Geometry check sheet. Reference: the model listing, model coordinates, mm. A direction names the side the tool comes from. Round coordinates to 2 decimals unless told otherwise and drop trailing zeros. Write each loop counter-clockwise with the first axis right and the second up, starting at its lowest first coordinate (ties: lowest second). Pieces come first, ordered by that corner, then holes. Notation, with made-up numbers: M -10,53 L 37,53 A27 ccw 37,86 Z; hole C -7,31.25 d9. An arc over 180 degrees is marked long. One line per item, written item: value. Start each with the question number.
1. Section check D-D (y = -2). Record the boundary of the cut face in (x, z).
2. Release check for a two-part mould opening along Z. For faces 1 (the flat face through (32, -2, 33)), 2 (the flat face through (41, -28.6, 17)), 3 (the flat face through (1.479, -19.529, 12.122)) record: pulls with the +Z half, pulls with the -Z half, needs draft (parallel to the pull), parting line crosses it, or undercut.
3. Access from +Z, -Z, +X, -X, +Y, -Y to the whole of each face (thin tool, end or side, straight path). Record for faces 4 (the flat face through (0, -21, 13)), 5 (the flat face through (54, -22.6, 17)), 6 (the flat face through (1.479, -8.922, 12.271)), 7 (the flat face through (65, -5, 17)).
4. Section check B-B (z = 29). Record the boundary of the cut face in (x, y).
5. Section check C-C (x = 47). Record the boundary of the cut face in (y, z), and give its area (3 significant figures).
6. Depth check by flat-ended pin: P1, Ø3, axis at y = -14.3, z = 17.5, coming from the +X side; P2, Ø6, axis at y = -17.5, z = 7.5, coming from the +X side; P3, Ø3, axis at y = -3.5, z = 27.5, coming from the +X side. Enter the tip coordinate at first touch or a pass-through.
7. Section check A-A (x = 7). Record the boundary of the cut face in (y, z), and give its area (3 significant figures).
8. Scan lines: probe 1 along Z at (x, y) = (9.25, -14.3); probe 2 along Y at (x, z) = (32.5, 29); probe 3 along X at (y, z) = (-19.5, 26.5). Record each from-to range of solid material in increasing order. Write a range as [from, to].
from build123d import *

# Parameters (mm, degrees)
EXTRUDE_1_DEPTH     = 35
CUT_EXTRUDE_2_DEPTH = 3
SKETCH_4_R          = 2.5
CUT_EXTRUDE_3_DEPTH = 15
CHAMFER_2_SIZE      = 4
CHAMFER_3_SIZE      = 4
CHAMFER_4_SIZE      = 4
CHAMFER_4_SIZE2     = 15
CHAMFER_5_SIZE      = 15
CHAMFER_5_SIZE2     = 4


with BuildPart() as part:
    # Эскиз2 → Бобышка-Вытянуть1 (new body)
    with BuildSketch(Plane.XY):
        Polygon((0, 0), (65, 0), (65, -6), (15, -6), (15, -22.6), (95, -22.6), (95, -28.6), (0, -28.6), align=None)
    extrude(amount=EXTRUDE_1_DEPTH)

    # Эскиз3 → Вырез-Вытянуть2 (cut)
    with BuildSketch(Plane.ZY):
        Polygon((6.893398282, -14.3), (17.5, -24.906601718), (28.106601718, -14.3), (17.5, -3.693398282), align=None)
    extrude(amount=-CUT_EXTRUDE_2_DEPTH, mode=Mode.SUBTRACT)

    # Эскиз4 → Вырез-Вытянуть3 (cut)
    with BuildSketch(Plane.ZY):
        with Locations(Location((17.5, -14.3, 0), (0, 0, 270))):
            Circle(SKETCH_4_R)
    extrude(amount=-CUT_EXTRUDE_3_DEPTH, mode=Mode.SUBTRACT)

    # Фаска2
    chamfer_2_edges = [part.edges().sort_by_distance(p)[0] for p in [
        (15, -11.8, 17.5),
    ]]
    chamfer(chamfer_2_edges, length=CHAMFER_2_SIZE)

    # Фаска3
    chamfer_3_edges = [part.edges().sort_by_distance(p)[0] for p in [
        (47.5, -28.6, 0),
        (32.5, 0, 35),
        (32.5, 0, 0),
        (47.5, -28.6, 35),
    ]]
    chamfer(chamfer_3_edges, length=CHAMFER_3_SIZE)

    # Фаска4
    chamfer_4_edges = [part.edges().sort_by_distance(p)[0] for p in [
        (65, 0, 17.5),
    ]]
    chamfer_4_side = [part.faces().sort_by_distance(p)[0] for p in [
        (65, -3.137457045, 17.5),
    ]]
    chamfer(chamfer_4_edges, length=CHAMFER_4_SIZE, length2=CHAMFER_4_SIZE2, reference=chamfer_4_side[0])

    # Фаска5
    chamfer_5_edges = [part.edges().sort_by_distance(p)[0] for p in [
        (95, -28.6, 17.5),
    ]]
    chamfer_5_side = [part.faces().sort_by_distance(p)[0] for p in [
        (47.5, -28.6, 17.5),
    ]]
    chamfer(chamfer_5_edges, length=CHAMFER_5_SIZE, length2=CHAMFER_5_SIZE2, reference=chamfer_5_side[0])


solid = part.part
Result sheet:
1. outline: M 0,2 L 57.5,2 L 57.5,33 L 0,33 Z
2. face 1: pulls with the +Z half
2. face 2: needs draft
2. face 3: undercut
3. face 4: +Z, -Z, -X, +Y, -Y
3. face 5: +Z, -Z, +X
3. face 6: -X
3. face 7: +Z, -Z, +X, +Y
4. outline: M 0,-28.6 L 80,-28.6 L 95,-24.6 L 95,-22.6 L 15,-22.6 L 15,-6 L 65,-6 L 65,-4 L 50,0 L 0,0 Z
5. outline: M -28.6,4 L -24.6,0 L -22.6,0 L -22.6,35 L -24.6,35 L -28.6,31 Z; M -6,0 L -4,0 L 0,4 L 0,31 L -4,35 L -6,35 Z
5. area: 388 mm2
6. P1: passes through
6. P2: stops at x = 15
6. P3: stops at x = 65
7. outline: M -28.6,4 L -24.6,0 L -4,0 L 0,4 L 0,31 L -4,35 L -24.6,35 L -28.6,31 Z; hole C -14.3,17.5 d5
7. area: 949 mm2
8. probe 1: z = [0, 15], [20, 35]
8. probe 2: y = [-28.6, -22.6], [-6, 0]
8. probe 3: x = [0, 15]
